from build123d import *

# Parameters (mm, degrees)
BOSS_EXTRUDE1_DEPTH     = 18
SKETCH2_R               = 7.5
SKETCH2_W               = 9
SKETCH2_H               = 5.5
CUT_EXTRUDE1_DEPTH      = 51.410812332
FILLET1_R               = 5
FILLET2_R               = 0.5
FILLET3_R               = 2
FILLET4_R               = 2.75
CUT_EXTRUDE2_DEPTH      = 15
SKETCH7_R               = 1.6
CUT_EXTRUDE3_DEPTH      = 10
SKETCH8_R               = 2.35
CUT_EXTRUDE4_DEPTH      = 5
SKETCH9_R               = 2.5
CUT_EXTRUDE5_DEPTH      = 0.5
MIRROR3_COPY_1_SKETCH_R = 1.6
MIRROR3_COPY_1_DEPTH    = 10
MIRROR3_COPY_2_SKETCH_R = 2.35
MIRROR3_COPY_2_DEPTH    = 5
MIRROR3_COPY_3_SKETCH_R = 2.5
MIRROR3_COPY_3_DEPTH    = 0.5
BOSS_EXTRUDE2_DEPTH     = 27
SKETCH11_W              = 11
SKETCH11_H              = 20
CUT_EXTRUDE6_DEPTH      = 21.2
SKETCH12_W              = 11
SKETCH12_H              = 3.7
CUT_EXTRUDE7_DEPTH      = 12.5
FILLET5_R               = 10
CUT_EXTRUDE8_REACH      = 67.133
SKETCH13_W              = 11
SKETCH13_H              = 19.8
FILLET6_R               = 10
SKETCH14_W              = 11
SKETCH14_H              = 7.4
CUT_EXTRUDE9_DEPTH      = 12.5
SKETCH15_R              = 2.75
BOSS_EXTRUDE3_DEPTH     = 0.8
BOSS_EXTRUDE3_TAPER     = 30
SKETCH16_W              = 14
SKETCH16_H              = 6.815
CUT_EXTRUDE10_DEPTH     = 0.8
SKETCH19_R              = 2.75
BOSS_EXTRUDE4_DEPTH     = 0.8
BOSS_EXTRUDE4_TAPER     = 30
FILLET7_R               = 2


with BuildPart() as part:
    # Sketch1 → Boss-Extrude1 (new body)
    with BuildSketch(Plane.XY):
        with BuildLine():
            Line((-17.5, 17.5), (-31.5, 3.5))
            Line((-31.5, 3.5), (-31.5, -3.5))
            Line((-31.5, -3.5), (-17.5, -17.5))
            Line((-17.5, -17.5), (17.5, -17.5))
            Line((17.5, -17.5), (31.5, -3.5))
            Line((31.5, -3.5), (31.5, 3.5))
            Line((31.5, 3.5), (17.5, 17.5))
            Line((17.5, 17.5), (13.560660172, 17.5))
            Line((13.560660172, 17.5), (17.25, 13.810660172))
            Line((17.25, 13.810660172), (17.25, 9.845660172))
            Line((17.25, 9.845660172), (21.927294091, 5.168366081))
            ThreePointArc((21.927294091, 5.168366081), (23.518574248, -5.09926529), (21.043225857, 4.991774143))
            Line((21.043225857, 4.991774143), (16.5, 9.535))
            Line((16.5, 9.535), (16.5, 13.5))
            Line((16.5, 13.5), (12.5, 17.5))
            Line((12.5, 17.5), (-12.5, 17.5))
            Line((-12.5, 17.5), (-16.5, 13.5))
            Line((-16.5, 13.5), (-16.5, 9.535))
            Line((-16.5, 9.535), (-21.043225857, 4.991774143))
            ThreePointArc((-21.043225857, 4.991774143), (-23.518574248, -5.09926529), (-21.927294091, 5.168366081))
            Line((-21.927294091, 5.168366081), (-17.25, 9.845660172))
            Line((-17.25, 9.845660172), (-17.25, 13.810660172))
            Line((-17.25, 13.810660172), (-13.560660172, 17.5))
            Line((-13.560660172, 17.5), (-17.5, 17.5))
        make_face()
    extrude(amount=BOSS_EXTRUDE1_DEPTH)

    # Sketch2 → Cut-Extrude1 (cut, through all)
    with BuildSketch(Plane(origin=(0, 17.5, 0), x_dir=(1, 0, 0), z_dir=(0, 1, 0))):
        Circle(SKETCH2_R)
        with Locations((-5.5, -15.25)):
            Rectangle(SKETCH2_W, SKETCH2_H)
    extrude(amount=-CUT_EXTRUDE1_DEPTH, mode=Mode.SUBTRACT)

    # Fillet1
    fillet1_edges = [part.edges().sort_by_distance(p)[0] for p in [
        (17.5, 17.5, 9),
        (31.5, 3.5, 9),
        (31.5, -3.5, 9),
        (17.5, -17.5, 9),
        (-17.5, -17.5, 9),
        (-31.5, -3.5, 9),
        (-31.5, 3.5, 9),
        (-17.5, 17.5, 9),
    ]]
    fillet(fillet1_edges, radius=FILLET1_R)

    # Fillet2
    fillet2_edges = [part.edges().sort_by_distance(p)[0] for p in [
        (-13.560660172, 17.5, 9),
        (-21.927294091, 5.168366081, 9),
        (-21.043225857, 4.991774143, 9),
        (21.043225857, 4.991774143, 9),
        (21.927294091, 5.168366081, 9),
        (13.560660172, 17.5, 9),
    ]]
    fillet(fillet2_edges, radius=FILLET2_R)

    # Fillet3
    fillet3_edges = [part.edges().sort_by_distance(p)[0] for p in [
        (-17.25, 9.845660172, 9),
        (17.25, 9.845660172, 9),
    ]]
    fillet(fillet3_edges, radius=FILLET3_R)

    # Fillet4
    fillet4_edges = [part.edges().sort_by_distance(p)[0] for p in [
        (-16.5, 9.535, 9),
        (16.5, 9.535, 9),
    ]]
    fillet(fillet4_edges, radius=FILLET4_R)

    # Sketch4 → Cut-Revolve1 (revolve, cut)
    with BuildSketch(Plane(origin=(0, 0, 6), x_dir=(-1, 0, 0), z_dir=(0, 0, -1))):
        Polygon((23.439696962, 11.560303038), (25.561017306, 9.438982694), (23.439696962, 7.317662351), (22.555813485, 8.201545827), (14.070532111, -0.283735547), (12.833095244, 0.95370132), align=None)
    cut_revolve1 = revolve(axis=Axis((-23.439696962, 11.560303038, 6), (0.7071067811865471, -0.707106781186548, 0)), mode=Mode.SUBTRACT)

    # Sketch6 → Cut-Extrude2 (cut)
    with BuildSketch(Plane(origin=(-6.893398282, 6.893398282, 0), x_dir=(0, 0, 1), z_dir=(-0.7071067811865471, 0.707106781186548, 0))):
        Polygon((3.425, -9.886676943), (6, -11.373353886), (8.575, -9.886676943), (8.575, -6.913323057), (6, -5.426646114), (3.425, -6.913323057), align=None)
    cut_extrude2 = extrude(amount=-CUT_EXTRUDE2_DEPTH, mode=Mode.SUBTRACT)

    # Mirror1: Cut-Revolve1, Cut-Extrude2 across plane
    add(cut_revolve1.mirror(Plane(origin=(0, 0, 0), x_dir=(0, 0, 1), z_dir=(1, 0, 0))), mode=Mode.SUBTRACT)
    add(cut_extrude2.mirror(Plane(origin=(0, 0, 0), x_dir=(0, 0, 1), z_dir=(1, 0, 0))), mode=Mode.SUBTRACT)

    # Sketch7 → Cut-Extrude3 (cut)
    with BuildSketch(Plane(origin=(0, 0, 0), x_dir=(-1, 0, 0), z_dir=(0, 0, -1))):
        with Locations((-12.5, 12.5)):
            Circle(SKETCH7_R)
    cut_extrude3 = extrude(amount=-CUT_EXTRUDE3_DEPTH, mode=Mode.SUBTRACT)

    # Sketch8 → Cut-Extrude4 (cut)
    with BuildSketch(Plane(origin=(0, 0, 0), x_dir=(-1, 0, 0), z_dir=(0, 0, -1))):
        with Locations((-12.5, 12.5)):
            Circle(SKETCH8_R)
    cut_extrude4 = extrude(amount=-CUT_EXTRUDE4_DEPTH, mode=Mode.SUBTRACT)

    # Sketch9 → Cut-Extrude5 (cut)
    with BuildSketch(Plane(origin=(0, 0, 0), x_dir=(-1, 0, 0), z_dir=(0, 0, -1))):
        with Locations((-12.5, 12.5)):
            Circle(SKETCH9_R)
    cut_extrude5 = extrude(amount=-CUT_EXTRUDE5_DEPTH, mode=Mode.SUBTRACT)

    # Mirror2: Cut-Extrude3, Cut-Extrude4, Cut-Extrude5 across plane
    add(cut_extrude3.mirror(Plane.ZX), mode=Mode.SUBTRACT)
    add(cut_extrude4.mirror(Plane.ZX), mode=Mode.SUBTRACT)
    add(cut_extrude5.mirror(Plane.ZX), mode=Mode.SUBTRACT)

    # Mirror3: Cut-Extrude3, Cut-Extrude4, Cut-Extrude5 across plane
    add(cut_extrude3.mirror(Plane(origin=(0, 0, 0), x_dir=(0, 0, 1), z_dir=(1, 0, 0))), mode=Mode.SUBTRACT)
    add(cut_extrude4.mirror(Plane(origin=(0, 0, 0), x_dir=(0, 0, 1), z_dir=(1, 0, 0))), mode=Mode.SUBTRACT)
    add(cut_extrude5.mirror(Plane(origin=(0, 0, 0), x_dir=(0, 0, 1), z_dir=(1, 0, 0))), mode=Mode.SUBTRACT)

    # Mirror3 copy 1 sketch → Mirror3 copy 1 (cut)
    with BuildSketch(Plane(origin=(0, 0, 0), x_dir=(1, 0, 0), z_dir=(0, 0, -1))):
        with Locations((-12.5, 12.5)):
            Circle(MIRROR3_COPY_1_SKETCH_R)
    extrude(amount=-MIRROR3_COPY_1_DEPTH, mode=Mode.SUBTRACT)

    # Mirror3 copy 2 sketch → Mirror3 copy 2 (cut)
    with BuildSketch(Plane(origin=(0, 0, 0), x_dir=(1, 0, 0), z_dir=(0, 0, -1))):
        with Locations((-12.5, 12.5)):
            Circle(MIRROR3_COPY_2_SKETCH_R)
    extrude(amount=-MIRROR3_COPY_2_DEPTH, mode=Mode.SUBTRACT)

    # Mirror3 copy 3 sketch → Mirror3 copy 3 (cut)
    with BuildSketch(Plane(origin=(0, 0, 0), x_dir=(1, 0, 0), z_dir=(0, 0, -1))):
        with Locations((-12.5, 12.5)):
            Circle(MIRROR3_COPY_3_SKETCH_R)
    extrude(amount=-MIRROR3_COPY_3_DEPTH, mode=Mode.SUBTRACT)

    # Sketch10 → Boss-Extrude2 (add)
    with BuildSketch(Plane.XY.offset(18)):
        Polygon((12.5, 17.5), (-12.5, 17.5), (-16.5, 13.5), (-16.5, -13.5), (-12.5, -17.5), (12.5, -17.5), (16.5, -13.5), (16.5, 13.5), align=None)
    extrude(amount=BOSS_EXTRUDE2_DEPTH)

    # Sketch11 → Cut-Extrude6 (cut)
    with BuildSketch(Plane(origin=(0, 17.5, 0), x_dir=(1, 0, 0), z_dir=(0, 1, 0))):
        with Locations((5.5, -22.5)):
            Rectangle(SKETCH11_W, SKETCH11_H)
    extrude(amount=-CUT_EXTRUDE6_DEPTH, mode=Mode.SUBTRACT)

    # Sketch12 → Cut-Extrude7 (cut)
    with BuildSketch(Plane(origin=(0, 0, 32.5), x_dir=(-1, 0, 0), z_dir=(0, 0, -1))):
        with Locations((-5.5, 1.85)):
            Rectangle(SKETCH12_W, SKETCH12_H)
        Polygon((-11, -3.7), (0, -3.7), (0, -3.591245546), (0, 0), (-11, 0), align=None)
    extrude(amount=-CUT_EXTRUDE7_DEPTH, mode=Mode.SUBTRACT)

    # Fillet5
    fillet5_edges = [part.edges().sort_by_distance(p)[0] for p in [
        (5.5, -3.7, 12.5),
    ]]
    fillet(fillet5_edges, radius=FILLET5_R)

    # Cut-Extrude8: up to this face of the body (flat: up to its plane)
    cut_extrude8_end = Plane(part.part.faces().sort_by_distance((5.5, 3.7, 38.75))[0])
    # Sketch13 → Cut-Extrude8 (cut, up to the picked face)
    with BuildSketch(Plane.XZ.offset(17.5), mode=Mode.PRIVATE) as cut_extrude8_sk1:
        with Locations((-5.5, 35.1)):
            Rectangle(SKETCH13_W, SKETCH13_H)
    cut_extrude8_tool1 = split(extrude(cut_extrude8_sk1.sketch, amount=-CUT_EXTRUDE8_REACH, mode=Mode.PRIVATE), bisect_by=cut_extrude8_end, keep=Keep.BOTH, mode=Mode.PRIVATE)
    add(cut_extrude8_tool1.solids().sort_by(Axis((-5.5, -17.5, 35.1), (0, 1, 0)))[0], mode=Mode.SUBTRACT)

    # Fillet6
    # the kernel refuses this fillet: 10 mm, written as the material it adds along each edge
    with BuildSketch(Plane(origin=(25, 3.7, 25.2), x_dir=(0, 0, 1), z_dir=(-1, 0, 0))) as fillet6_piece_1_section:
        with BuildLine():
            CenterArc((FILLET6_R, -FILLET6_R), FILLET6_R, 90, 90)
            Line((0, -FILLET6_R), (0, 0))
            Line((0, 0), (FILLET6_R, 0))
        make_face()
    fillet6_piece_1 = extrude(amount=36, mode=Mode.PRIVATE)
    fillet6_piece_1 = split(fillet6_piece_1, bisect_by=Plane(origin=(5.5, 3.588944861, 32.5), z_dir=(0, 0, 1)), keep=Keep.TOP, mode=Mode.PRIVATE)
    fillet6_piece_1 = split(fillet6_piece_1, bisect_by=Plane(origin=(11, 3.588944861, 33.172467691), z_dir=(-1, 0, 0)), keep=Keep.TOP, mode=Mode.PRIVATE)
    add(fillet6_piece_1)
    with BuildSketch(Plane(origin=(0, 3.7, 25.2), x_dir=(0, 0, 1), z_dir=(-1, 0, 0))) as fillet6_piece_2:
        with BuildLine():
            CenterArc((FILLET6_R, -FILLET6_R), FILLET6_R, 90, 90)
            Line((0, -FILLET6_R), (0, 0))
            Line((0, 0), (FILLET6_R, 0))
        make_face()
    extrude(amount=11)

    # Sketch14 → Cut-Extrude9 (cut)
    with BuildSketch(Plane.XY.offset(45)):
        with Locations((5.5, 0)):
            Rectangle(SKETCH14_W, SKETCH14_H)
    extrude(amount=-CUT_EXTRUDE9_DEPTH, mode=Mode.SUBTRACT)

    # Sketch15 → Boss-Extrude3 (add)
    with BuildSketch(Plane(origin=(-11, 0, 0), x_dir=(0, 0, -1), z_dir=(1, 0, 0))):
        with Locations((-35.23, -6.365)):
            Circle(SKETCH15_R)
    extrude(amount=BOSS_EXTRUDE3_DEPTH, taper=BOSS_EXTRUDE3_TAPER)

    # Sketch16 → Cut-Extrude10 (cut)
    with BuildSketch(Plane.ZY):
        with Locations((38, -7.1075)):
            Rectangle(SKETCH16_W, SKETCH16_H)
    extrude(amount=-CUT_EXTRUDE10_DEPTH, mode=Mode.SUBTRACT)

    # Sketch17 → Cut-Revolve2 (revolve, cut)
    with BuildSketch(Plane.XY.offset(35.23)):
        Polygon((-16.5, -6.365), (-16.5, -3.265), (-13.5, -3.265), (-13.5, -4.865), (11.5, -4.865), (11.5, -4.115), (16, -4.115), (16, -3.865), (16.5, -3.865), (16.5, -6.365), align=None)
    revolve(axis=Axis((31.947720378, -6.365, 35.23), (-1, 0, 0)), mode=Mode.SUBTRACT)

    # Sketch19 → Boss-Extrude4 (add)
    with BuildSketch(Plane.ZY.offset(-11)):
        with Locations((22.5, 6.365)):
            Circle(SKETCH19_R)
    boss_extrude4 = extrude(amount=BOSS_EXTRUDE4_DEPTH, taper=BOSS_EXTRUDE4_TAPER)

    # Mirror4: Boss-Extrude4 across plane
    add(boss_extrude4.mirror(Plane(origin=(5.5, 0, 0), x_dir=(0, 0, 1), z_dir=(1, 0, 0))))

    # Sketch20 → Cut-Revolve3 (revolve, cut)
    with BuildSketch(Plane.XY.offset(22.5), mode=Mode.PRIVATE) as cut_revolve3_sk:
        Polygon((16.5, 6.365), (16.5, 9.465), (13.5, 9.465), (13.5, 7.865), (-11.5, 7.865), (-11.5, 8.615), (-16, 8.615), (-16, 8.865), (-16.5, 8.865), (-16.5, 6.365), align=None)
    revolve(cut_revolve3_sk.sketch.rotate(Axis((11, 6.365, 22.5), (-1, 0, 0)), 90), axis=Axis((11, 6.365, 22.5), (-1, 0, 0)), mode=Mode.SUBTRACT)

    # Fillet7
    fillet7_edges = [part.edges().sort_by_distance(p)[0] for p in [
        (16.5, -13.5, 31.5),
        (12.5, -17.5, 31.5),
        (-12.5, -17.5, 31.5),
        (-16.5, -13.5, 31.5),
        (-16.5, 13.5, 22.5),
        (-12.5, 17.5, 22.5),
        (12.5, 17.5, 22.5),
        (16.5, 13.5, 22.5),
    ]]
    fillet(fillet7_edges, radius=FILLET7_R)


solid = part.part
Geometry check sheet. Reference: the model listing, model coordinates, mm. A direction names the side the tool comes from. Give positions to 0.01 mm unless a question says otherwise; leave off trailing zeros. Order: outer loops, then holes, each group sorted by start corner. A loop starts at its lowest first (then second) coordinate and runs counter-clockwise, first axis right, second up. Notation, with made-up numbers: M -28.5,-37 L -24.5,-37 A21 cw -24.5,-4 Z; hole C 49,-30.75 d1. An arc over 180 degrees is marked long. Use a Markdown table: item, result.
Item 1: Tool access check on faces 4 (the flat face through (-10, -2, 3.425)), 5 (the flat face through (0.8, -7, 38)), 6 (the flat face through (15, 15, 22)), 7 (the cylindrical face through (-14.1, 12.57, 7.46)). Record the directions out of +Z, -Z, +X, -X, +Y, -Y that give a thin tool (end or side, any length) a straight path to the whole face; none if there is none.
Answers follow:
| item | result |
|---|---|
| face 4 | none |
| face 5 | +Z |
| face 6 | +Z, -Z |
| face 7 | -Z |
Item 2: Depth check by flat-ended pin: P1, Ø3.5, axis at y = 11.5, z = 9, coming from the +X side; P2, Ø1, axis at y = -6, z = 30.5, coming from the +X side; P3, Ø1.9, axis at x = 12.5, y = 12.5, coming from the -Z side. Enter the tip coordinate at first touch or a pass-through.
Answers follow:
| item | result |
|---|---|
| P1 | stops at x = 25.25 |
| P2 | stops at x = 16.5 |
| P3 | stops at z = 10 |
Item 3: Draft check along Y on faces 1 (the flat face through (-15, -15, 31)), 2 (the flat face through (0, 4, 45)), 3 (the cylindrical face through (-23.56, -5.09, 8.87)). Enter one of: +Y half, -Y half, draft (parallel to the pull), parting line (faces both ways), or undercut.
Answers follow:
| item | result |
|---|---|
| face 1 | -Y half |
| face 2 | draft |
| face 3 | undercut |
Item 4: Material ranges on line 1 along X through (y, z) = (3, 23); line 2 along Z through (x, y) = (8, -6); line 3 along X through (y, z) = (0, 4), recorded low to high.
Answers follow:
| item | result |
|---|---|
| line 1 | x = -16.5 to 0, 11 to 16.5 |
| line 2 | z = 0 to 3.45, 8.55 to 33.78, 36.68 to 45 |
| line 3 | x = -31.5 to -27.7, -17.3 to -13.79, -9.31 to -6.34, 6.34 to 9.31, 13.79 to 17.3, 27.7 to 31.5 |
Item 5: Section check B-B (z = 42.5). Record the cut outline in (x, y) (3 decimals), and give its area (3 significant figures).
Answers follow:
| item | result |
|---|---|
| outline | M -16.5,-12.672 A2 ccw -15.914,-14.086 L -13.086,-16.914 A2 ccw -11.672,-17.5 L -11,-17.5 L -11,3.7 L 11,3.7 L 11,-3.7 L 0.8,-3.7 L 0.8,-10.515 L 0,-10.515 L 0,-17.5 L 11.672,-17.5 A2 ccw 13.086,-16.914 L 15.914,-14.086 A2 ccw 16.5,-12.672 L 16.5,12.672 A2 ccw 15.914,14.086 L 13.086,16.914 A2 ccw 11.672,17.5 L -11.672,17.5 A2 ccw -13.086,16.914 L -15.914,14.086 A2 ccw -16.5,12.672 Z |
| area | 802 mm2 |
Item 6: Section check A-A (x = 9). Record the cut outline in (y, z) (3 decimals), and give its area (3 significant figures).
Answers follow:
| item | result |
|---|---|
| outline | M -17.5,0 L 17.5,0 L 17.5,12.5 L 6.3,12.5 A10 cw -3.7,22.5 L -3.7,45 L -17.5,45 Z; M 3.7,32.5 L 17.5,32.5 L 17.5,45 L 3.7,45 Z; hole C -6.365,35.23 d3; hole M -7.084,6 L -4.982,3.425 L -0.777,3.425 L 1.326,6 L -0.777,8.575 L -4.982,8.575 Z |
| area | 1,040 mm2 |
Item 7: Section check C-C (x = 26.5). Record the cut outline in (y, z).
Answers follow:
| item | result |
|---|---|
| outline | M -8.5,0 L -3.32,0 L -3.32,18 L -8.5,18 Z; M 3.32,0 L 8.5,0 L 8.5,18 L 3.32,18 Z |
